from build123d import *

# Parameters (mm, degrees)
SKETCH1_R           = 9.906
SKETCH1_R_2         = 12.7
BOSS_EXTRUDE1_DEPTH = 5.6896
FILLET1_R           = 2.54


with BuildPart() as part:
    # Sketch1 → Boss-Extrude1 (new body)
    with BuildSketch(Plane.XY):
        with BuildLine():
            ThreePointArc((13.085798561, 50.8), (0, 63.885798561), (-13.085798561, 50.8))
            Line((-13.085798561, 50.8), (-15.879798561, 0))
            ThreePointArc((-15.879798561, 0), (0, -16.777187541), (15.879798561, 0))
            Line((15.879798561, 0), (13.085798561, 50.8))
        make_face()
        with BuildLine():
            Line((-12.197482286, 9.136685717), (-10.290993585, 43.800116641))
            ThreePointArc((-10.290993585, 43.800116641), (0, 38.354), (10.290993585, 43.800116641))
            Line((10.290993585, 43.800116641), (12.197482286, 9.136685717))
            ThreePointArc((12.197482286, 9.136685717), (0, 15.24), (-12.197482286, 9.136685717))
        make_face(mode=Mode.SUBTRACT)
        with Locations((0, 50.8)):
            Circle(SKETCH1_R, mode=Mode.SUBTRACT)
        Circle(SKETCH1_R_2, mode=Mode.SUBTRACT)
    extrude(amount=BOSS_EXTRUDE1_DEPTH)

    # Fillet1
    fillet1_edges = [part.edges().sort_by_distance(p)[0] for p in [
        (-10.290993585, 43.800116641, 2.8448),
        (-12.197482286, 9.136685717, 2.8448),
        (12.197482286, 9.136685717, 2.8448),
        (10.290993585, 43.800116641, 2.8448),
    ]]
    fillet(fillet1_edges, radius=FILLET1_R)


solid = part.part
The listing builds one solid part. Answer for the finished solid, in the listing's coordinates (mm). A direction names the side the tool comes from. Coordinates: 2 decimals unless noted, no trailing zeros. Write each loop counter-clockwise with the first axis right and the second up, starting at its lowest first coordinate (ties: lowest second). Pieces come first, ordered by that corner, then holes. Notation, with made-up numbers: (-10.5, 10.25) - (35.5, 10.25) arc R26 ccw to (35.5, 34.25) - close; hole circle Ø4 at (45.5, 62.25). An arc over 180 degrees is marked (long way). Answer as CSV lines item,"result".
1. Find section A-A (x = 0). Give the vertices of the cut face in (y, z), plus the area to 3 significant figures.
Computed values:
outline,"(-16.78, 0) - (-12.7, 0) - (-12.7, 5.69) - (-16.78, 5.69) - close; (12.7, 0) - (15.24, 0) - (15.24, 5.69) - (12.7, 5.69) - close; (38.35, 0) - (40.89, 0) - (40.89, 5.69) - (38.35, 5.69) - close; (60.71, 0) - (63.89, 0) - (63.89, 5.69) - (60.71, 5.69) - close"
area,"70.2 mm²"
2. Find section D-D (x = -4). Give the vertices of the cut face in (y, z).
Computed values:
outline,"(-16.27, 0) - (-12.05, 0) - (-12.05, 5.69) - (-16.27, 5.69) - close; (12.05, 0) - (14.71, 0) - (14.71, 5.69) - (12.05, 5.69) - close; (39.01, 0) - (41.74, 0) - (41.74, 5.69) - (39.01, 5.69) - close; (59.86, 0) - (63.26, 0) - (63.26, 5.69) - (59.86, 5.69) - close"
3. A tool of negligible diameter and unlimited length cuts with its end or side. For faces 5 (the cylindrical face through (0.12, 15.24, 2.8)), 6 (the flat face through (0, 15, 5.69)), from which of +Z, -Z, +X, -X, +Y, -Y can it reach the whole face along a straight path? Write none if from no direction.
Computed values:
face 5,"+Z, -Z"
face 6,"+Z, +X, -X, +Y, -Y"
4. Given P1, Ø2, axis at x = -4.5, z = 2, coming from the -Y side; P2, Ø1.5, axis at x = -9, z = 1, coming from the +Y side, each flat-ended and moving along its own axis, determine where each tip first touches the part or whether it passes through.
Computed values:
P1,"stops at y = -16.39"
P2,"stops at y = 60.96"
5. Straight lines are drawn through the part: line 1 (Y direction, x = 0, z = 3.65); line 2 (Y direction, x = 10, z = 1.35); line 3 (Y direction, x = -9, z = 5.05). For each, find the intervals that lie inside material, in ascending order. Write a range as [from, to].
Computed values:
line 1,"y = [-16.78, -12.7], [12.7, 15.24], [38.35, 40.89], [60.71, 63.89]"
line 2,"y = [-13.24, -7.83], [7.83, 12.69], [39.8, 59.24]"
line 3,"y = [-13.99, -8.96], [8.96, 12.62], [40.52, 46.66], [54.94, 60.3]"
6. Determine the mould class of faces 1 (the flat face through (11.218, 26.952, 2.805)), 2 (the cylindrical face through (0.288, 63.883, 2.805)), 3 (the cylindrical face through (9.25, 40.407, 2.885)), 4 (the flat face through (0, 15, 0)) for opening direction Y: +Y half, -Y half, draft (parallel to the pull), parting line (faces both ways), or undercut.
Computed values:
face 1,"undercut"
face 2,"+Y half"
face 3,"undercut"
face 4,"draft"
7. Find section B-B (z = 0.85). Give the vertices of the cut face in (x, y).
Computed values:
outline,"(-15.88, 0) arc R15.9 ccw (long way) to (15.88, 0) - (13.09, 50.8) arc R13.09 ccw to (-13.09, 50.8) - close; hole circle Ø25.4 at (0, 0); hole (-11.86, 15.28) arc R2.54 ccw to (-7.99, 12.98) arc R15.24 cw to (7.99, 12.98) arc R2.54 ccw to (11.86, 15.28) - (10.59, 38.3) arc R2.54 ccw to (6.69, 40.31) arc R12.45 cw to (-6.69, 40.31) arc R2.54 ccw to (-10.59, 38.3) - close; hole circle Ø19.81 at (0, 50.8)"
8. Find section C-C (y = 5). Give the vertices of the cut face in (x, z), plus the area to 3 significant figures.
Computed values:
outline,"(-15.6, 0) - (-11.67, 0) - (-11.67, 5.69) - (-15.6, 5.69) - close; (11.67, 0) - (15.6, 0) - (15.6, 5.69) - (11.67, 5.69) - close"
area,"44.7 mm²"
